```python
from build123d import *

# Parameters (mm, degrees)
SKETCH047_W     = 105.8
SKETCH047_H     = 25.7
SKETCH047_W_2   = 20.1
SKETCH047_H_2   = 20.1
PAD026_DEPTH    = 6
SKETCH043_R     = 45.225
SKETCH043_R_2   = 40.225
PAD027_DEPTH    = 6
POCKET028_DEPTH = 6
POCKET026_DEPTH = 6
FILLET011_R     = 1
SKETCH049_W     = 25.7
SKETCH049_H     = 25.7
SKETCH049_W_2   = 20.1
SKETCH049_H_2   = 20.1
PAD023_DEPTH    = 10
SKETCH045_R     = 2.75
POCKET031_DEPTH = 105.8
SKETCH042_R     = 2.75
POCKET029_DEPTH = 2.8
FILLET010_R     = 1
PAD024_DEPTH    = 36.6
PAD025_DEPTH    = 2.8
SKETCH048_W     = 139.326154
SKETCH048_H     = 62.3
POCKET027_DEPTH = 61
SKETCH044_W     = 139.326154
SKETCH044_H     = 18
SKETCH044_H_2   = 13
POCKET030_DEPTH = 45
SKETCH052_W     = 20.1
SKETCH052_H     = 20.1
SKETCH052_R     = 2.75
PAD029_DEPTH    = 2.8


with BuildPart() as part:
    # Sketch047 → Pad026 (new body)
    with BuildSketch(Plane.XY):
        with Locations((52.9, 12.85)):
            Rectangle(SKETCH047_W, SKETCH047_H)
        with Locations((12.85, 12.85)):
            Rectangle(SKETCH047_W_2, SKETCH047_H_2, mode=Mode.SUBTRACT)
        with Locations((92.95, 12.85)):
            Rectangle(SKETCH047_W_2, SKETCH047_H_2, mode=Mode.SUBTRACT)
    extrude(amount=PAD026_DEPTH)

    # Sketch043 → Pad027 (join)
    with BuildSketch(Plane.XY):
        with Locations((52.9, -37.955)):
            Circle(SKETCH043_R)
        with Locations((52.9, -37.955)):
            Circle(SKETCH043_R_2, mode=Mode.SUBTRACT)
    extrude(amount=PAD027_DEPTH)

    # Pad027 Face25 → Pocket028 (cut)
    with BuildSketch(Plane(origin=(52.9, 0.910232, 6), x_dir=(0, 1, 0), z_dir=(0, 0, 1))):
        with BuildLine():
            ThreePointArc((-0.910232, -13.321734), (1.359768, 0), (-0.910232, 13.321734))
            Line((-0.910232, 13.321734), (-0.910232, -13.321734))
        make_face()
    extrude(amount=-POCKET028_DEPTH, mode=Mode.SUBTRACT)

    # Sketch050 → Pocket026 (cut)
    with BuildSketch(Plane.XY):
        with BuildLine():
            Line((52.9, -37.955), (94.041911, -66.762877))
            ThreePointArc((11.758089, -66.762877), (52.9, -88.18), (94.041911, -66.762877))
            Line((52.9, -37.955), (11.758089, -66.762877))
        make_face()
    extrude(amount=POCKET026_DEPTH, mode=Mode.SUBTRACT)

    # Fillet011
    fillet011_edges = [part.edges().sort_by_distance(p)[0] for p in [
        (19.949609, -61.027112, 3),
        (85.850391, -61.027112, 3),
    ]]
    fillet(fillet011_edges, radius=FILLET011_R)

    # Sketch049 (on Face11 of Fillet011) → Pad023 (join)
    with BuildSketch(Plane(origin=(0, 0, 0), x_dir=(1, 0, 0), z_dir=(0, 0, -1))):
        with Locations((12.85, -12.85)):
            Rectangle(SKETCH049_W, SKETCH049_H)
        with Locations((12.85, -12.85)):
            Rectangle(SKETCH049_W_2, SKETCH049_H_2, mode=Mode.SUBTRACT)
        with Locations((92.95, -12.85)):
            Rectangle(SKETCH049_W, SKETCH049_H)
        with Locations((92.95, -12.85)):
            Rectangle(SKETCH049_W_2, SKETCH049_H_2, mode=Mode.SUBTRACT)
    extrude(amount=PAD023_DEPTH)

    # Sketch045 (on Face27 of Pad023) → Pocket031 (cut)
    with BuildSketch(Plane(origin=(0, 0, 0), x_dir=(0, -1, 0), z_dir=(-1, 0, 0))):
        with Locations((-12.85, -5)):
            Circle(SKETCH045_R)
    extrude(amount=-POCKET031_DEPTH, mode=Mode.SUBTRACT)

    # Sketch042 (on Face13 of Pocket031) → Pocket029 (cut)
    with BuildSketch(Plane.XZ):
        with Locations((12.85, -5)):
            Circle(SKETCH042_R)
        with Locations((92.95, -5)):
            Circle(SKETCH042_R)
    extrude(amount=-POCKET029_DEPTH, mode=Mode.SUBTRACT)

    # Fillet010
    fillet010_edges = [part.edges().sort_by_distance(p)[0] for p in [
        (103, 12.85, -10),
        (92.95, 2.8, -10),
        (82.9, 12.85, -10),
        (22.9, 12.85, -10),
        (12.85, 2.8, -10),
        (2.8, 12.85, -10),
        (0, 0, -5),
        (0, 0, 3),
        (105.8, 0, -5),
        (105.8, 0, 3),
    ]]
    fillet(fillet010_edges, radius=FILLET010_R)

    # Sketch046 (on Face12 of Fillet010) → Pad024 (join)
    with BuildSketch(Plane(origin=(0, 25.7, 0), x_dir=(-1, 0, 0), z_dir=(0, 1, 0))):
        with BuildLine():
            Line((12.1, 6), (-117.9, 6))
            ThreePointArc((-117.9, 6), (-121.340012, 1.51689), (-122.563077, -4))
            ThreePointArc((-122.563077, -4), (-52.9, -73.663077), (16.763077, -4))
            ThreePointArc((16.763077, -4), (15.540012, 1.51689), (12.1, 6))
        make_face()
    extrude(amount=PAD024_DEPTH)

    # Pad024 Face4 → Pad025 (add)
    with BuildSketch(Plane(origin=(52.9, 25.7, -32.391454), x_dir=(-1, 0, 0), z_dir=(0, -1, 0))):
        with BuildLine():
            ThreePointArc((65, -38.391454), (68.440012, -33.908343), (69.663077, -28.391454))
            ThreePointArc((69.663077, -28.391454), (0, 41.271623), (-69.663077, -28.391454))
            ThreePointArc((-69.663077, -28.391454), (-68.440012, -33.908343), (-65, -38.391454))
            Line((-65, -38.391454), (-52.9, -38.391454))
            Line((-52.9, -38.391454), (-52.9, -32.391454))
            Line((-52.9, -32.391454), (-52.9, -22.391454))
            Line((-52.9, -22.391454), (-27.2, -22.391454))
            Line((-27.2, -22.391454), (-27.2, -32.391454))
            Line((-27.2, -32.391454), (27.2, -32.391454))
            Line((27.2, -32.391454), (27.2, -22.391454))
            Line((27.2, -22.391454), (52.9, -22.391454))
            Line((52.9, -22.391454), (52.9, -32.391454))
            Line((52.9, -32.391454), (52.9, -38.391454))
            Line((52.9, -38.391454), (65, -38.391454))
        make_face()
    extrude(amount=PAD025_DEPTH)

    # Sketch048 → Pocket027 (cut)
    with BuildSketch(Plane.XY.offset(-49)):
        with Locations((52.9, 31.15)):
            Rectangle(SKETCH048_W, SKETCH048_H)
    extrude(amount=-POCKET027_DEPTH, mode=Mode.SUBTRACT)

    # Sketch044 (on Face28 of Pocket027) → Pocket030 (cut)
    with BuildSketch(Plane(origin=(0, 0, -49), x_dir=(1, 0, 0), z_dir=(0, 0, -1))):
        with Locations((52.9, -34.7)):
            Rectangle(SKETCH044_W, SKETCH044_H)
        with Locations((52.9, -53)):
            Rectangle(SKETCH044_W, SKETCH044_H_2)
    extrude(amount=-POCKET030_DEPTH, mode=Mode.SUBTRACT)

    # Sketch052 (on Face5 of Pocket030) → Pad029 (join)
    with BuildSketch(Plane.XY.offset(6)):
        with Locations((12.85, 12.85)):
            Rectangle(SKETCH052_W, SKETCH052_H)
        with Locations((12.85, 12.85)):
            Circle(SKETCH052_R, mode=Mode.SUBTRACT)
        with Locations((92.95, 12.85)):
            Rectangle(SKETCH052_W, SKETCH052_H)
        with Locations((92.95, 12.85)):
            Circle(SKETCH052_R, mode=Mode.SUBTRACT)
    extrude(amount=-PAD029_DEPTH)


with BuildPart() as part_1:
    # Body007 placement: moved
    add(part.part.moved(Location((800, 0, 40))))


solid = part_1.part
```
Could you check a few things on this model? Use its own coordinates, in mm. A direction names the side the tool comes from. Coordinates: 2 decimals unless noted, no trailing zeros. Write each loop counter-clockwise with the first axis right and the second up, starting at its lowest first coordinate (ties: lowest second). Pieces come first, ordered by that corner, then holes. Notation, with made-up numbers: (34, 68) -> (85, 68) arc R23 ccw to (85, 79) -> close; hole circle Ø8 at (76, 86). An arc over 180 degrees is marked (long way). Write item = value, one per line. Start each with the question number.
(1) I want a section at A-A (y = -14). Please give me the cut outline in (x, z).
(2) We'd pull the mould along Y, two halves only. Please class faces 1 (the face through (891, 1, 30)), 2 (the face through (854, 62.3, 19)), 3 (the face through (890.6, 10.8, 43.2)), 4 (the face through (801.38, 13.208, 37.727)): released by +Y, released by -Y, zero draft, split by the parting line, or undercut.
(3) I want a section at C-C (z = 11.5). Please give me the cut outline in (x, y), plus the area to 3 significant figures.
(4) Which directions (+Z, -Z, +X, -X, +Y, -Y) give clear straight access to the entire face, cutting with the end or side of a thin tool? Please do faces 5 (the face through (811, 1, 30)), 6 (the face through (822.9, 13, 39)), 7 (the face through (852, 28, 46)), 8 (the face through (852, 43.7, 13)).
(5) Will these pins go through, and if not, where does the flat tip stop? pin 1 (22.5 mm diameter, centred on x = 862, z = 13.5, fed in from -Y); pin 2 (6.5 mm diameter, centred on y = 12.85, z = 35, fed in from -X); pin 3 (10.5 mm diameter, centred on x = 885.5, y = 55, fed in from -Z); pin 4 (12 mm diameter, centred on x = 837.5, y = -4, fed in from -Z).
(6) I want a section at B-B (x = 806). Please give me the cut outline in (y, z), plus the area to 3 significant figures.
(7) I need wall thicknesses on line 1 (Y direction, x = 859.5, z = 35); line 2 (X direction, y = 12, z = 44); line 3 (Y direction, x = 878.5, z = 42). Which ranges of each line are inside material? Lowest first, please. Write a range as [from, to].
(8) I want a section at D-D (y = 12.85). Give the number of separate pieces and of enclosed holes in the cut face, plus the area to 3 significant figures.
Result set:
q1.outline = (814.54, 40) -> (820.59, 40) -> (820.59, 46) -> (814.54, 46) -> close; (885.21, 40) -> (891.26, 40) -> (891.26, 46) -> (885.21, 46) -> close
q2.face_1 = zero draft
q2.face_2 = released by +Y
q2.face_3 = undercut
q2.face_4 = undercut
q3.outline = (787.69, 22.9) -> (918.11, 22.9) -> (918.11, 25.7) -> (787.69, 25.7) -> close; (787.69, 43.7) -> (918.11, 43.7) -> (918.11, 46.5) -> (787.69, 46.5) -> close; (787.69, 59.5) -> (918.11, 59.5) -> (918.11, 62.3) -> (787.69, 62.3) -> close
q3.area = 1,100 mm2
q4.face_5 = -Z, +X, -X, -Y
q4.face_6 = -Z
q4.face_7 = +Z, +X, -X, +Y, -Y
q4.face_8 = -Z, +X, -X
q5.pin_1 = 22.9
q5.pin_2 = 800
q5.pin_3 = -9
q5.pin_4 = 40
q6.outline = (0, 30) -> (1.8, 30) arc R1 ccw to (2.8, 31) -> (2.8, 43.2) -> (22.9, 43.2) -> (22.9, -9) -> (25.7, -9) -> (25.7, 36) -> (43.7, 36) -> (43.7, -9) -> (46.5, -9) -> (46.5, 36) -> (59.5, 36) -> (59.5, -9) -> (62.3, -9) -> (62.3, 46) -> (0, 46) -> close
q6.area = 873 mm2
q7.line_1 = [22.9, 25.7], [43.7, 46.5], [59.5, 62.3]
q7.line_2 = [800, 810.23], [815.47, 890.33], [895.57, 905.8]
q7.line_3 = [-6.93, -0.67], [0, 62.3]
q8.separate_pieces = 7
q8.enclosed_holes = 0
q8.area = 525 mm2
